```python
from build123d import *

# Parameters (mm, degrees)
F0_R          = 285.75
F1_DEPTH      = 431.8
F2_W          = 381
F2_H          = 635
F3_DEPTH      = 452.12
F4_T          = -2.54
F5_W          = 104.14
F5_H          = 104.14
F6_DEPTH      = 285.751
F6_DEPTH_BACK = 285.751


with BuildPart() as f1:
    # F0 (on Front) → F1 (new body, symmetric)
    with BuildSketch(Plane.XZ):
        Circle(F0_R)
    extrude(amount=F1_DEPTH, both=True)

    # F2 (on Top) → F3 (cut)
    with BuildSketch(Plane.XY):
        Rectangle(F2_W, F2_H)
    extrude(amount=F3_DEPTH, mode=Mode.SUBTRACT)

    # F4
    f4_openings = [f1.faces().sort_by_distance(p)[0] for p in [
        (0, 317.5, 132.295443),
        (-190.5, 0, 106.492737),
        (0, 0, 0),
        (0, -317.5, 132.295443),
        (190.5, 0, 106.492737),
    ]]
    offset(amount=F4_T, openings=f4_openings)

    # F5 (on Right) → F6 (cut, two sides)
    with BuildSketch(Plane.YZ) as f6_sk:
        Rectangle(F5_W, F5_H)
    extrude(amount=-F6_DEPTH, mode=Mode.SUBTRACT)
    extrude(f6_sk.sketch, amount=F6_DEPTH_BACK, mode=Mode.SUBTRACT)


solid = f1.part
```
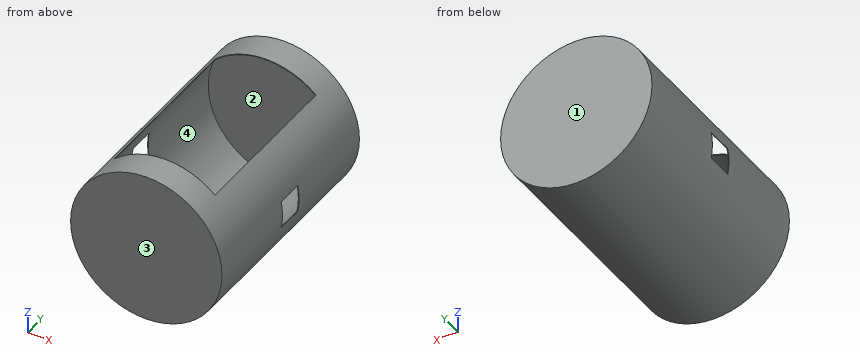
Model file for the job. Use its own axes, mm. Face numbers are marked on the shaded views. Round coordinates to 2 decimals unless told otherwise and drop trailing zeros. Write each loop counter-clockwise with the first axis right and the second up, starting at its lowest first coordinate (ties: lowest second). Pieces come first, ordered by that corner, then holes. Notation, with made-up numbers: (88.5, -36) - (100.5, -36) arc R35 ccw to (100.5, 2) - close; hole circle Ø7 at (3.25, 58). An arc over 180 degrees is marked (long way). One line per item, written item: value.
(1) Cut at B-B, the plane x = 0. Give the cut face in (y, z).
Values follow:
outline: (-431.8, -285.75) - (431.8, -285.75) - (431.8, 285.75) - (317.5, 285.75) - (317.5, 283.21) - (429.26, 283.21) - (429.26, -283.21) - (-429.26, -283.21) - (-429.26, 283.21) - (-317.5, 283.21) - (-317.5, 285.75) - (-431.8, 285.75) - close
(2) Two-plate mould, pull along Y, no slides. Class the marked faces 1, 2, 3 and 4: pulls with the +Y half, pulls with the -Y half, needs draft (parallel to the pull), parting line crosses it, or undercut.
Values follow:
face 1: pulls with the +Y half
face 2: undercut
face 3: pulls with the -Y half
face 4: undercut
(3) Wall check: probe 1 along Y at (x, z) = (164.5, 75.5); probe 2 along X at (y, z) = (142, 0); probe 3 along Z at (x, y) = (0, 242). Give the ranges that are in metal, low to high.
Values follow:
probe 1: y = -431.8 to -429.26, 429.26 to 431.8
probe 2: x = -285.75 to -283.21, 283.21 to 285.75
probe 3: z = -285.75 to -283.21
(4) Drop flat-ended pins along their axis: P1, Ø10, axis at x = -147.5, y = 8, coming from the +Z side; P2, Ø1, axis at x = -214, y = -67, coming from the -Z side; P3, Ø1.5, axis at x = -132.5, y = -124.5, coming from the +Z side. Give the stop position or say it passes through.
Values follow:
P1: stops at z = -238.65
P2: stops at z = -189.92
P3: stops at z = -249.9
(5) Cut at A-A, the plane z = 0. Give the cut face in (x, y).
Values follow:
outline: (-285.75, -431.8) - (285.75, -431.8) - (285.75, -52.07) - (283.21, -52.07) - (283.21, -429.26) - (-283.21, -429.26) - (-283.21, -52.07) - (-285.75, -52.07) - close; (-285.75, 52.07) - (-283.21, 52.07) - (-283.21, 429.26) - (283.21, 429.26) - (283.21, 52.07) - (285.75, 52.07) - (285.75, 431.8) - (-285.75, 431.8) - close
